Verification items for the finished model (mm, model axes). A direction names the side the tool comes from. Coordinates: 2 decimals unless noted, no trailing zeros. Order: outer loops, then holes, each group sorted by start corner. A loop starts at its lowest first (then second) coordinate and runs counter-clockwise, first axis right, second up. Notation, with made-up numbers: (11.25, 49.5) -> (35.25, 49.5) arc R23 cw to (35.25, 80.5) -> close; hole circle Ø9 at (71, 15.5). An arc over 180 degrees is marked (long way). Answer as CSV lines item,"result".
```python
from build123d import *

# Parameters (mm, degrees)
F1_DEPTH = 50.8
F2_R     = 12.7
F3_DEPTH = 5.08
F4_SIZE  = 5.08
F5_R     = 3.679261


with BuildPart() as f1:
    # F0 (on Front) → F1 (new body)
    with BuildSketch(Plane.XZ):
        Polygon((0, 25.4), (0, 0), (76.2, 0), (76.2, 69.394091), align=None)
    extrude(amount=F1_DEPTH)

    # F2 (on face) → F3 (cut)
    with BuildSketch(Plane.XZ.offset(50.8)):
        with Locations((55.88, 30.48)):
            Circle(F2_R)
    extrude(amount=-F3_DEPTH, mode=Mode.SUBTRACT)

    # F4
    f4_edges = [f1.edges().sort_by_distance(p)[0] for p in [
        (0, 0, 12.7),
        (38.1, 0, 0),
        (76.2, 0, 34.697045),
        (38.1, 0, 47.397045),
    ]]
    chamfer(f4_edges, length=F4_SIZE)

    # F5
    f5_edges = [f1.edges().sort_by_distance(p)[0] for p in [
        (38.1, -50.8, 0),
    ]]
    fillet(f5_edges, radius=F5_R)


solid = f1.part
```
Item 1: Section check D-D, the plane x = 45. Record the boundary of the cut face in (y, z), plus the area to 3 significant figures.
Answer list:
outline,"(-50.8, 3.68) arc R3.68 ccw to (-47.12, 0) -> (-5.08, 0) -> (0, 5.08) -> (0, 45.51) -> (-5.08, 51.38) -> (-50.8, 51.38) -> (-50.8, 37.03) -> (-45.72, 37.03) -> (-45.72, 23.93) -> (-50.8, 23.93) -> close"
area,"2,510 mm2"
Item 2: Depth check by flat-ended pin: pin 1 Ø10 at (x, y) = (17, -25.5) entering from +Z; pin 2 Ø12.5 at (x, z) = (56.5, 35) entering from -Y; pin 3 Ø1 at (y, z) = (-39.5, 27.5) entering from -X. Enter the tip coordinate at first touch or a pass-through.
Answer list:
pin 1,"z = 38.1"
pin 2,"y = -45.72"
pin 3,"x = 2.77"
Item 3: Thickness scan on line 1 (Y direction, x = 52, z = 25); line 2 (Z direction, x = 55, y = -49); line 3 (X direction, y = -49, z = 30). Record the ranges inside material, lowest first.
Answer list:
line 1,"-45.72 to 0"
line 2,"0.52 to 17.81, 43.15 to 57.15"
line 3,"7.97 to 43.19, 68.57 to 76.2"
Item 4: Section check A-A, the plane x = 16.5. Record the boundary of the cut face in (y, z), plus the area to 3 significant figures.
Answer list:
outline,"(-50.8, 3.68) arc R3.68 ccw to (-47.12, 0) -> (-5.08, 0) -> (0, 5.08) -> (0, 29.06) -> (-5.08, 34.93) -> (-50.8, 34.93) -> close"
area,"1,740 mm2"
Item 5: Release check for a two-part mould opening along Z. For faces 3 (the flat face through (38.633, -27.62, 47.705)), 4 (the flat face through (56, -45.72, 31)), 5 (the cylindrical face through (38.633, -49.751, 1.106)) record: +Z half, -Z half, draft (parallel to the pull), parting line (faces both ways), or undercut.
Answer list:
face 3,"+Z half"
face 4,"undercut"
face 5,"-Z half"
Item 6: Section check B-B, the plane z = 30.48. Record the boundary of the cut face in (x, y).
Answer list:
outline,"(8.8, -50.8) -> (43.18, -50.8) -> (43.18, -45.72) -> (68.58, -45.72) -> (68.58, -50.8) -> (76.2, -50.8) -> (76.2, -5.08) -> (71.12, 0) -> (18.96, 0) -> (8.8, -5.08) -> close"
Item 7: Tool access check on faces 1 (the cylindrical face through (45.802, -48.296, 22.752)), 2 (the flat face through (37.57, -2.5, 2.58)). Record the directions out of +Z, -Z, +X, -X, +Y, -Y that give a thin tool (end or side, any length) a straight path to the whole face; none if there is none.
Answer list:
face 1,"-Y"
face 2,"-Z, +X, -X, +Y"
Item 8: Section check C-C, the plane y = -22.5. Record the boundary of the cut face in (x, z).
Answer list:
outline,"(0, 0) -> (76.2, 0) -> (76.2, 69.39) -> (0, 25.4) -> close"
